Verification items for the finished model (mm, model axes). A direction names the side the tool comes from. Round coordinates to 2 decimals unless told otherwise and drop trailing zeros. Loops run counter-clockwise (first coordinate to the right, second up) from the corner with the lowest first, then second, coordinate; pieces in that order, holes last. Notation, with made-up numbers: (38, 58) - (65, 58) arc R21 ccw to (65, 62) - close; hole circle Ø8 at (86, 48.5). An arc over 180 degrees is marked (long way). Use CSV: the item, a comma, the result in double quotes.
```python
from build123d import *

# Parameters (mm, degrees)
F1_DEPTH = 32
F2_R     = 6.5
F3_DEPTH = 88.001
F5_DEPTH = 88.001
F6_R     = 5.5
F7_DEPTH = 13.001
F8_DEPTH = 13.001


with BuildPart() as f1:
    # F0 (on Front) → F1 (new body)
    with BuildSketch(Plane.XZ):
        Polygon((0, 13), (0, 0), (39, 0), (39, 17), (74, 17), (74, 0), (113, 0), (113, 13), (88, 13), (88, 64), (69, 64), (69, 30), (44, 30), (44, 64), (25, 64), (25, 13), align=None)
    extrude(amount=-F1_DEPTH)

    # F2 (on face) → F3 (cut, through all)
    with BuildSketch(Plane.YZ.offset(88)):
        with Locations((16, 46)):
            Circle(F2_R)
    extrude(amount=-F3_DEPTH, mode=Mode.SUBTRACT)

    # F4 (on face) → F5 (cut, through all)
    with BuildSketch(Plane.YZ.offset(88)):
        with BuildLine():
            ThreePointArc((0, 60.790067), (6.535448, 63.059972), (13.389709, 64))
            Line((13.389709, 64), (0, 64))
            Line((0, 64), (0, 60.790067))
        make_face()
        with BuildLine():
            ThreePointArc((16, 64), (24.274438, 62.687848), (32, 59.446899))
            Line((32, 59.446899), (32, 64))
            Line((32, 64), (16, 64))
        make_face()
    extrude(amount=-F5_DEPTH, mode=Mode.SUBTRACT)

    # F6 (on face) → F7 (cut, through all)
    with BuildSketch(Plane.XY.offset(13)):
        Polygon((0, 10), (0, 0), (10, 0), align=None)
        Polygon((113, 10), (103, 0), (113, 0), align=None)
        with Locations((100, 19)):
            Circle(F6_R)
    extrude(amount=-F7_DEPTH, mode=Mode.SUBTRACT)

    # F6 (on face) → F8 (cut, through all)
    with BuildSketch(Plane.XY.offset(13)):
        with Locations((13, 19)):
            Circle(F6_R)
    extrude(amount=-F8_DEPTH, mode=Mode.SUBTRACT)


solid = f1.part
```
1) Cross-section at A-A, the plane z = 7. Record the cut outline in (x, y).
Returned:
outline,"(0, 10) - (10, 0) - (39, 0) - (39, 32) - (0, 32) - close; (74, 0) - (103, 0) - (113, 10) - (113, 32) - (74, 32) - close; hole circle Ø11 at (13, 19); hole circle Ø11 at (100, 19)"
2) Cross-section at B-B, the plane x = 13. Record the cut outline in (y, z), then the cut area to 3 significant figures.
Returned:
outline,"(0, 0) - (13.5, 0) - (13.5, 13) - (0, 13) - close; (24.5, 0) - (32, 0) - (32, 13) - (24.5, 13) - close"
area,"273 mm²"
3) Cross-section at D-D, the plane x = 85. Record the cut outline in (y, z), then the cut area to 3 significant figures.
Returned:
outline,"(0, 0) - (32, 0) - (32, 59.45) arc R35 ccw to (16, 64) - (13.39, 64) arc R35 ccw to (0, 60.79) - close; hole circle Ø13 at (16, 46)"
area,"1,870 mm²"
4) Thickness scan on probe 1 along Z at (x, y) = (40, 16); probe 2 along X at (y, z) = (5, 56.5); probe 3 along Z at (x, y) = (33.25, 16). Record the ranges inside material, lowest first. Write a range as [from, to].
Returned:
probe 1,"z = [17, 39.5], [52.5, 64]"
probe 2,"x = [25, 44], [69, 88]"
probe 3,"z = [0, 39.5], [52.5, 64]"
5) Cross-section at C-C, the plane z = 46. Record the cut outline in (x, y).
Returned:
outline,"(25, 0) - (44, 0) - (44, 9.5) - (25, 9.5) - close; (25, 22.5) - (44, 22.5) - (44, 32) - (25, 32) - close; (69, 0) - (88, 0) - (88, 9.5) - (69, 9.5) - close; (69, 22.5) - (88, 22.5) - (88, 32) - (69, 32) - close"
6) Access from +Z, -Z, +X, -X, +Y, -Y to the whole of each face (thin tool, end or side, straight path). Record for faces 4 (the face through (44, 16, 39)), 5 (the face through (19, 16, 0)), 6 (the face through (78.633, 10.842, 42.045)), 7 (the face through (56, 16, 17)), 8 (the face through (25, 16, 39)).
Returned:
face 4,"+Z, +Y, -Y"
face 5,"-Z, +X, -X, +Y, -Y"
face 6,"+X, -X"
face 7,"-Z, +Y, -Y"
face 8,"+Z, -X, +Y, -Y"
7) Mould release check, pull along X, two halves, no side actions. Record for faces 1 (the face through (113, 21, 6)), 2 (the face through (94.505, 19.242, 6.591)), 3 (the face through (34.63, 24.16, 62.72)): +X half, -X half, draft (parallel to the pull), parting line (faces both ways), or undercut.
Returned:
face 1,"+X half"
face 2,"undercut"
face 3,"draft"
8) Gauge pin test, flat ends, axial feed: pin 1 Ø2 at (y, z) = (19.5, 38) entering from +X; pin 2 Ø2 at (y, z) = (17.5, 22.5) entering from -X; pin 3 Ø12.5 at (x, y) = (99.5, 15.5) entering from +Z. Record the tip position at first contact, or that the pin passes through.
Returned:
pin 1,"stops at x = 88"
pin 2,"stops at x = 25"
pin 3,"stops at z = 13"
